from build123d import *

# Parameters (mm, degrees)
SKETCH1_R           = 25
BOSS_EXTRUDE1_DEPTH = 2
SKETCH2_R           = 1.05
SKETCH2_R_2         = 0.79375
CUT_EXTRUDE1_DEPTH  = 3
SKETCH4_R           = 2.05
CUT_EXTRUDE3_DEPTH  = 3
SKETCH7_R           = 0.79375
SKETCH7_R_2         = 0.28575
BOSS_EXTRUDE2_DEPTH = 8.64
FILLET1_R           = 1
FILLET2_R           = 1
FILLET3_R           = 1
FILLET4_R           = 1


with BuildPart() as part:
    # Sketch1 → Boss-Extrude1 (new body)
    with BuildSketch(Plane(origin=(0, 0, 0), x_dir=(1, 0, 0), z_dir=(0, 1, 0))):
        Circle(SKETCH1_R)
    extrude(amount=BOSS_EXTRUDE1_DEPTH)

    # Sketch2 → Cut-Extrude1 (cut, through all)
    with BuildSketch(Plane(origin=(0, 2, 0), x_dir=(1, 0, 0), z_dir=(0, 1, 0))):
        with Locations((-2.066368974, 7.209723938)):
            Circle(SKETCH2_R)
        with Locations((7.209723938, 2.066368974)):
            Circle(SKETCH2_R)
        with Locations((2.066368974, -7.209723938)):
            Circle(SKETCH2_R)
        with Locations((-7.209723938, -2.066368974)):
            Circle(SKETCH2_R)
        with Locations((-3.636901173, -6.559188201)):
            Circle(SKETCH2_R_2)
        with Locations((-6.559188201, 3.636901173)):
            Circle(SKETCH2_R_2)
        with Locations((3.636901173, 6.559188201)):
            Circle(SKETCH2_R_2)
        with Locations((6.559188201, -3.636901173)):
            Circle(SKETCH2_R_2)
    extrude(amount=-CUT_EXTRUDE1_DEPTH, mode=Mode.SUBTRACT)

    # Sketch4 → Cut-Extrude3 (cut, through all)
    with BuildSketch(Plane.XZ):
        with Locations((-18.488747294, 7.626678405)):
            Circle(SKETCH4_R)
        with Locations((-7.680642569, 18.466394605)):
            Circle(SKETCH4_R)
        with Locations((7.626678405, 18.488747294)):
            Circle(SKETCH4_R)
        with Locations((18.466394605, 7.680642569)):
            Circle(SKETCH4_R)
        with Locations((18.488747294, -7.626678405)):
            Circle(SKETCH4_R)
        with Locations((7.680642569, -18.466394605)):
            Circle(SKETCH4_R)
        with Locations((-7.626678405, -18.488747294)):
            Circle(SKETCH4_R)
        with Locations((-18.466394605, -7.680642569)):
            Circle(SKETCH4_R)
    extrude(amount=-CUT_EXTRUDE3_DEPTH, mode=Mode.SUBTRACT)

    # Sketch7 → Boss-Extrude2 (add)
    with BuildSketch(Plane(origin=(0, 0, 0), x_dir=(1, 0, 0), z_dir=(0, 1, 0))):
        with Locations((-3.636901173, -6.559188201)):
            Circle(SKETCH7_R)
        with Locations((-3.636901173, -6.559188201)):
            Circle(SKETCH7_R_2, mode=Mode.SUBTRACT)
        with Locations((6.559188201, -3.636901173)):
            Circle(SKETCH7_R)
        with Locations((6.559188201, -3.636901173)):
            Circle(SKETCH7_R_2, mode=Mode.SUBTRACT)
        with Locations((-6.559188201, 3.636901173)):
            Circle(SKETCH7_R)
        with Locations((-6.559188201, 3.636901173)):
            Circle(SKETCH7_R_2, mode=Mode.SUBTRACT)
        with Locations((3.636901173, 6.559188201)):
            Circle(SKETCH7_R)
        with Locations((3.636901173, 6.559188201)):
            Circle(SKETCH7_R_2, mode=Mode.SUBTRACT)
    extrude(amount=BOSS_EXTRUDE2_DEPTH)

    # Fillet1
    fillet1_edges = [part.edges().sort_by_distance(p)[0] for p in [
        (-7.352938201, 2, -3.636901173),
    ]]
    fillet(fillet1_edges, radius=FILLET1_R)

    # Fillet2
    fillet2_edges = [part.edges().sort_by_distance(p)[0] for p in [
        (-4.430651173, 2, 6.559188201),
    ]]
    fillet(fillet2_edges, radius=FILLET2_R)

    # Fillet3
    fillet3_edges = [part.edges().sort_by_distance(p)[0] for p in [
        (5.765438201, 2, 3.636901173),
    ]]
    fillet(fillet3_edges, radius=FILLET3_R)

    # Fillet4
    fillet4_edges = [part.edges().sort_by_distance(p)[0] for p in [
        (2.843151173, 2, -6.559188201),
    ]]
    fillet(fillet4_edges, radius=FILLET4_R)


solid = part.part
For this review, take the finished solid that the model builds, in its own axes (mm). A direction names the side the tool comes from. Round coordinates to 2 decimals unless told otherwise and drop trailing zeros. Loops run counter-clockwise (first coordinate to the right, second up) from the corner with the lowest first, then second, coordinate; pieces in that order, holes last. Notation, with made-up numbers: (-37.5, 28) - (-28.5, 28) arc R28 cw to (-28.5, 66) - close; hole circle Ø2 at (84, 61). An arc over 180 degrees is marked (long way). Put each result on its own line as item: value. Start each with the question number.
1. Mouldability with a two-part tool opening along Z and no side actions: class faces 1 (the cylindrical face through (5.93, 5.78, 4.12)), 2 (the cylindrical face through (3.036, 1.014, 7.612)), 3 (the flat face through (-4, 8.64, 7)) as +Z half, -Z half, draft (parallel to the pull), parting line (faces both ways), or undercut.
2. For faces 4 (the cylindrical face through (-9.25, 0.99, -19.74)), 5 (the flat face through (0, 2, 0)), list the 3-axis set-ups (+Z, -Z, +X, -X, +Y, -Y) from which the entire face can be reached by the end or side of a thin tool; tool diameter is ignored.
3. Consider section D-D on x = 0. State the section outline as (y, z) points.
4. For probe 1 along Y at (x, z) = (3.5, 18.5); probe 2 along Z at (x, y) = (18.5, 1.5); probe 3 along X at (y, z) = (1, 6), list the stretches that pass through material, from the lowest coordinate up. Write a range as [from, to].
5. Consider section A-A on y = 8. State the section outline as (x, z) points, plus the area to 3 significant figures.
6. Consider section B-B on x = 19. State the section outline as (y, z) points.
7. Consider section C-C on y = 1. State how many separate pieces and enclosed holes the cut face has, plus the area to 3 significant figures.
8. Insertion check: P1, Ø3.5, axis at x = -18.49, z = 7.63, coming from the +Y side; P2, Ø2, axis at y = 2, z = 18, coming from the -X side; P3, Ø5.5, axis at x = -18.47, z = -7.68, coming from the +Y side; P4, Ø2, axis at x = -10, y = 2, coming from the -Z side. Each pin has a flat end and moves straight along its axis. Give the tip position at first contact, or say it passes through.
Result sheet:
1. face 1: parting line
1. face 2: undercut
1. face 3: draft
2. face 4: +Y, -Y
2. face 5: +Y
3. outline: (0, -25) - (2, -25) - (2, 25) - (0, 25) - close
4. probe 1: [0, 2]
4. probe 2: [-16.82, -9.68], [-5.58, 5.63], [9.73, 16.82]
4. probe 3: [-24.27, -19.74], [-17.24, 17.29], [19.64, 24.27]
5. outline: circle Ø1.59 at (-6.56, -3.64); circle Ø1.59 at (-3.64, 6.56); circle Ø1.59 at (3.64, -6.56); circle Ø1.59 at (6.56, 3.64); hole circle Ø0.57 at (-6.56, -3.64); hole circle Ø0.57 at (-3.64, 6.56); hole circle Ø0.57 at (3.64, -6.56); hole circle Ø0.57 at (6.56, 3.64)
5. area: 6.89 mm^2
6. outline: (0, -16.25) - (2, -16.25) - (2, -9.61) - (0, -9.61) - close; (0, -5.64) - (2, -5.64) - (2, 5.7) - (0, 5.7) - close; (0, 9.66) - (2, 9.66) - (2, 16.25) - (0, 16.25) - close
7. separate pieces: 1
7. enclosed holes: 16
7. area: 1,840 mm^2
8. P1: through
8. P2: x = -18.33
8. P3: y = 2
8. P4: z = -23.32
